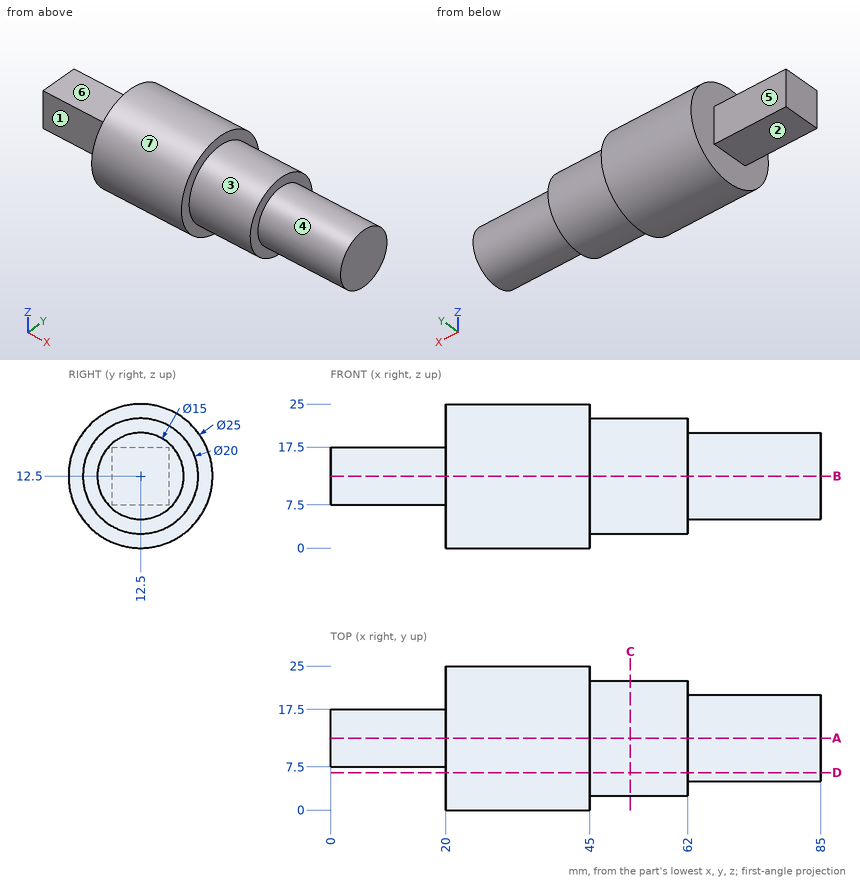
Source: three-view drawing plus pictorial views. Frame: mm from the lowest corner of the part. A direction names the side the tool comes from. Round coordinates to 2 decimals unless told otherwise and drop trailing zeros. Order: outer loops, then holes, each group sorted by start corner. A loop starts at its lowest first (then second) coordinate and runs counter-clockwise, first axis right, second up. Notation, with made-up numbers: (89.25, 23.5) -> (146.25, 23.5) arc R35 cw to (146.25, 62.5) -> close; hole circle Ø6 at (-12, 47). An arc over 180 degrees is marked (long way). Use one line per item in the form item = value. Start each with the question number.
1. Reachability of the marked faces 4, 5, 6 and 7 from +Z, -Z, +X, -X, +Y, -Y: full face, straight path, thin tool, end or side. Return the list, or none.
2. Pin query (flat end, axial travel): pin 1 Ø3 at (x, z) = (6, 12.5) entering from +Y; pin 2 Ø3 at (x, z) = (14.5, 10.5) entering from -Y; pin 3 Ø1 at (x, y) = (41.5, 13) entering from +Z; pin 4 Ø8 at (x, z) = (72, 3.5) entering from +Y. Return the tip coordinate at first contact, or that it passes through.
3. Line query: probe 1 along Y at (x, z) = (11.5, 15.75); probe 2 along X at (y, z) = (5.25, 18); probe 3 along Z at (x, y) = (41, 20). Output: solid intervals per line, ascending.
4. Cut plane D-D (y = 6.5). Return the cut outline in (x, z).
5. Cut plane C-C (x = 52). Return the cut outline in (y, z), then the cut area to 3 significant figures.
6. Cut plane A-A (y = 12.5). Return the cut outline in (x, z), then the cut area to 3 significant figures.
7. Draft query along Y for the marked faces 1, 2 and 3. Return one class per face: pulls with the +Y half, pulls with the -Y half, needs draft (parallel to the pull), parting line crosses it, or undercut.
Solution:
q1.face_4 = +X
q1.face_5 = +Z, -Z, -X, +Y
q1.face_6 = +Z, -X, +Y, -Y
q1.face_7 = +X, -X
q2.pin_1 = 17.5
q2.pin_2 = 7.5
q2.pin_3 = 25
q2.pin_4 = 18.09
q3.probe_1 = 7.5 to 17.5
q3.probe_2 = 20 to 62
q3.probe_3 = 2.5 to 22.5
q4.outline = (20, 1.53) -> (45, 1.53) -> (45, 4.5) -> (62, 4.5) -> (62, 8) -> (85, 8) -> (85, 17) -> (62, 17) -> (62, 20.5) -> (45, 20.5) -> (45, 23.47) -> (20, 23.47) -> close
q5.outline = circle Ø20 at (12.5, 12.5)
q5.area = 314 mm^2
q6.outline = (0, 7.5) -> (20, 7.5) -> (20, 0) -> (45, 0) -> (45, 2.5) -> (62, 2.5) -> (62, 5) -> (85, 5) -> (85, 20) -> (62, 20) -> (62, 22.5) -> (45, 22.5) -> (45, 25) -> (20, 25) -> (20, 17.5) -> (0, 17.5) -> close
q6.area = 1,510 mm^2
q7.face_1 = pulls with the -Y half
q7.face_2 = needs draft
q7.face_3 = parting line crosses it
